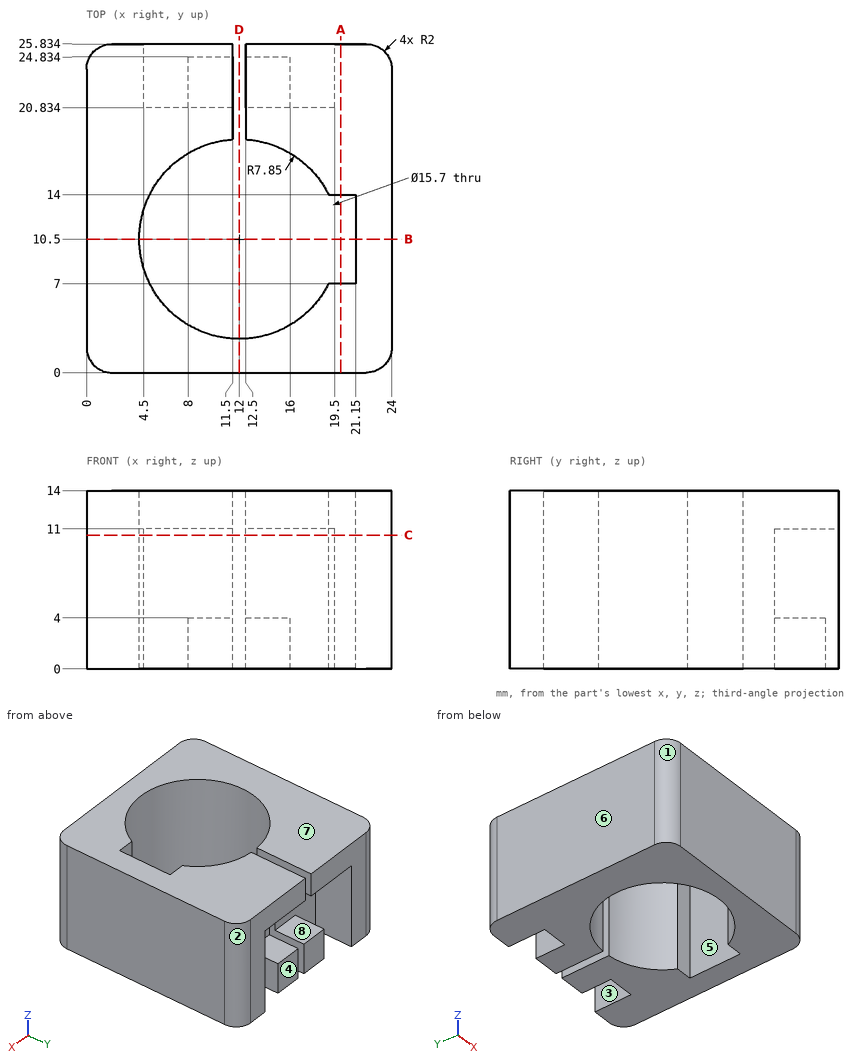
Geometry check sheet. Reference: drawing and pictorial views, mm from the part's lowest x, y, z. A direction names the side the tool comes from. Give positions to 0.01 mm unless a question says otherwise; leave off trailing zeros. Write each loop counter-clockwise with the first axis right and the second up, starting at its lowest first coordinate (ties: lowest second). Pieces come first, ordered by that corner, then holes. Notation, with made-up numbers: (-24.5, -36.5) - (-2.5, -36.5) arc R18 cw to (-2.5, -10.5) - close; hole circle Ø3 at (49, 81.5). An arc over 180 degrees is marked (long way). Use a Markdown table: item, result.
Q1. Section check A-A, the plane x = 20. Enter the section's corners in (y, z).
Computed:
| item | result |
|---|---|
| outline | (0, 0) - (7, 0) - (7, 14) - (0, 14) - close; (14, 0) - (25.83, 0) - (25.83, 14) - (14, 14) - close |
Q2. Go/stop test with flat-tipped pins: P1, Ø3, axis at x = 11.5, z = 2.5, coming from the +Y side; P2, Ø2, axis at x = 18, z = 4, coming from the +Y side. Record where each tip stops, or that it passes through.
Computed:
| item | result |
|---|---|
| P1 | stops at y = 24.83 |
| P2 | stops at y = 20.83 |
Q3. Section check C-C, the plane z = 10.5. Enter the section's corners in (x, y), then the cut area to 3 significant figures.
Computed:
| item | result |
|---|---|
| outline | (0, 2) arc R2 ccw to (2, 0) - (22, 0) arc R2 ccw to (24, 2) - (24, 23.83) arc R2 ccw to (22, 25.83) - (19.5, 25.83) - (19.5, 20.83) - (12.5, 20.83) - (12.5, 18.33) arc R7.85 cw to (19.03, 14) - (21.15, 14) - (21.15, 7) - (19.03, 7) arc R7.85 cw (long way) to (11.5, 18.33) - (11.5, 20.83) - (4.5, 20.83) - (4.5, 25.83) - (2, 25.83) arc R2 ccw to (0, 23.83) - close |
| area | 335 mm² |
Q4. Section check D-D, the plane x = 12. Enter the section's corners in (y, z), then the cut area to 3 significant figures.
Computed:
| item | result |
|---|---|
| outline | (0, 0) - (2.65, 0) - (2.65, 14) - (0, 14) - close |
| area | 37.1 mm² |
Q5. Draft check along X on the marked faces 1, 2 and 3. Enter one of: pulls with the +X half, pulls with the -X half, needs draft (parallel to the pull), parting line crosses it, or undercut.
Computed:
| item | result |
|---|---|
| face 1 | pulls with the -X half |
| face 2 | pulls with the +X half |
| face 3 | undercut |
Q6. Set-up check for the marked faces 4, 5, 6, 7 and 8: record each of +Z, -Z, +X, -X, +Y, -Y from which the full face is reachable in a straight line by a thin tool's end or side.
Computed:
| item | result |
|---|---|
| face 4 | -Z, +Y |
| face 5 | +Z, -Z |
| face 6 | +Z, -Z, -X, +Y, -Y |
| face 7 | +Z, +X, -X, +Y, -Y |
| face 8 | +Y |
Q7. Section check B-B, the plane y = 10.5. Enter the section's corners in (x, z).
Computed:
| item | result |
|---|---|
| outline | (0, 0) - (4.15, 0) - (4.15, 14) - (0, 14) - close; (21.15, 0) - (24, 0) - (24, 14) - (21.15, 14) - close |
Q8. Thickness scan on L1, parallel to X at y = 22.5, z = 3.75; L2, parallel to X at y = 10.75, z = 11.75; L3, parallel to Z at x = 19, y = 22.75. Record the ranges inside material, lowest first. Write a range as [from, to].
Computed:
| item | result |
|---|---|
| L1 | x = [0, 4.5], [8, 11.5], [12.5, 16], [19.5, 24] |
| L2 | x = [0, 4.15], [21.15, 24] |
| L3 | z = [11, 14] |
